```python
from build123d import *

# Parameters (mm, degrees)
F0_W      = 914.4
F0_H      = 1828.8
F1_DEPTH  = 25.4
F2_W      = 25.4
F2_H      = 25.4
F3_DEPTH  = 25.4
F4_W      = 25.4
F4_H      = 25.4
F5_DEPTH  = 25.4
F6_R      = 9.525
F7_DEPTH  = 25.4
F8_R      = 9.525
F9_DEPTH  = 25.4
F10_R     = 9.525
F11_DEPTH = 25.4
F12_R     = 9.525
F13_DEPTH = 25.4
F15_DEPTH = 25.4


with BuildPart() as f1:
    # F0 (on Front) → F1 (new body)
    with BuildSketch(Plane.XZ):
        Rectangle(F0_W, F0_H)
    extrude(amount=F1_DEPTH)

    # F2 (on face) → F3 (cut)
    with BuildSketch(Plane.XY.offset(914.4)):
        with Locations((-444.5, -12.7)):
            Rectangle(F2_W, F2_H)
        with Locations((444.5, -12.7)):
            Rectangle(F2_W, F2_H)
    extrude(amount=-F3_DEPTH, mode=Mode.SUBTRACT)

    # F4 (on face) → F5 (cut)
    with BuildSketch(Plane(origin=(0, 0, -914.4), x_dir=(1, 0, 0), z_dir=(0, 0, -1))):
        with Locations((-444.5, 12.7)):
            Rectangle(F4_W, F4_H)
        with Locations((444.5, 12.7)):
            Rectangle(F4_W, F4_H)
    extrude(amount=-F5_DEPTH, mode=Mode.SUBTRACT)

    # F6 (on face) → F7 (join)
    with BuildSketch(Plane.XY.offset(889)):
        with Locations((-444.5, -12.7)):
            Circle(F6_R)
    extrude(amount=F7_DEPTH)

    # F8 (on face) → F9 (join)
    with BuildSketch(Plane.XY.offset(889)):
        with Locations((444.5, -12.7)):
            Circle(F8_R)
    extrude(amount=F9_DEPTH)

    # F10 (on face) → F11 (join)
    with BuildSketch(Plane(origin=(0, 0, -889), x_dir=(1, 0, 0), z_dir=(0, 0, -1))):
        with Locations((-444.5, 12.7)):
            Circle(F10_R)
    extrude(amount=F11_DEPTH)

    # F12 (on face) → F13 (join)
    with BuildSketch(Plane(origin=(0, 0, -889), x_dir=(1, 0, 0), z_dir=(0, 0, -1))):
        with Locations((444.5, 12.7)):
            Circle(F12_R)
    extrude(amount=F13_DEPTH)

    # F14 (on face) → F15 (cut)
    with BuildSketch(Plane.XZ.offset(25.4)):
        Polygon((-377.825, 838.2), (-377.825, -914.4), (-323.85, -914.4), (-215.9, -914.4), (0, -914.4), (215.9, -914.4), (323.85, -914.4), (377.825, -914.4), (377.825, 838.2), align=None)
    extrude(amount=-F15_DEPTH, mode=Mode.SUBTRACT)


solid = f1.part
```
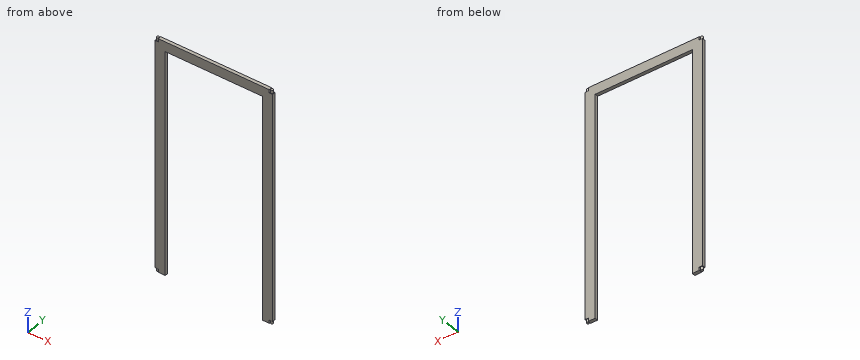
Source: CAD feature listing. Evaluate the final solid. Frame: model axes, mm. Give positions to 0.01 mm unless a question says otherwise; leave off trailing zeros. Write each loop counter-clockwise with the first axis right and the second up, starting at its lowest first coordinate (ties: lowest second). Pieces come first, ordered by that corner, then holes.
1. Material intervals for line 1 along X through (y, z) = (-18.75, 6) (3 decimals); line 2 along Z through (x, y) = (264.5, -9), sorted ascending.
2. Section query A-A (z = 457). Return the cut outline in (x, y) (3 decimals).
3. Section query C-C (x = 147). Return the cut outline in (y, z), then the cut area to 3 significant figures.
4. First-contact query: pin 1 (7.5 mm diameter, centred on x = 40, y = -11.5, fed in from -Z); pin 2 (7.5 mm diameter, centred on y = -17.5, z = 901, fed in from +X); pin 3 (7.5 mm diameter, centred on y = -15.5, z = 900, fed in from -X) (3 decimals). Flat tips, straight axial feed; report the tip coordinate or a pass-through.
Output values:
1. line 1: x = -457.2 to -377.825, 377.825 to 457.2
1. line 2: z = 838.2 to 914.4
2. outline: (-457.2, -25.4) - (-377.825, -25.4) - (-377.825, 0) - (-457.2, 0) - close; (377.825, -25.4) - (457.2, -25.4) - (457.2, 0) - (377.825, 0) - close
3. outline: (-25.4, 838.2) - (0, 838.2) - (0, 914.4) - (-25.4, 914.4) - close
3. area: 1,940 mm2
4. pin 1: stops at z = 838.2
4. pin 2: stops at x = 453.97
4. pin 3: stops at x = -454.025
